from build123d import *

# Parameters (mm, degrees)
SKETCH2_R           = 2
BOSS_EXTRUDE1_DEPTH = 6.7


with BuildPart() as part:
    # Sketch2 → Boss-Extrude1 (new body)
    with BuildSketch(Plane.XY):
        with BuildLine():
            Line((-4.409637173, -1.2), (-3.764514138, -0.899174188))
            ThreePointArc((-3.764514138, -0.899174188), (-3.582420347, -0.728223333), (-3.537232834, -0.482580436))
            ThreePointArc((-3.537232834, -0.482580436), (-3.57, 0), (-3.537232834, 0.482580436))
            ThreePointArc((-3.537232834, 0.482580436), (-3.582420347, 0.728223333), (-3.764514138, 0.899174188))
            Line((-3.764514138, 0.899174188), (-4.409637173, 1.2))
            ThreePointArc((-4.409637173, 1.2), (-4.294395277, 1.563032055), (-4.149323184, 1.915206806))
            Line((-4.149323184, 1.915206806), (-3.461763164, 1.730975654))
            ThreePointArc((-3.461763164, 1.730975654), (-3.212386135, 1.744883974), (-3.019874282, 1.904011377))
            ThreePointArc((-3.019874282, 1.904011377), (-2.734778662, 2.294751767), (-2.399480831, 2.6433675))
            ThreePointArc((-2.399480831, 2.6433675), (-2.276200264, 2.860586849), (-2.305807109, 3.108590435))
            Line((-2.305807109, 3.108590435), (-2.606632921, 3.75371347))
            ThreePointArc((-2.606632921, 3.75371347), (-2.285, 3.957736095), (-1.947494763, 4.134267063))
            Line((-1.947494763, 4.134267063), (-1.539214732, 3.55118275))
            ThreePointArc((-1.539214732, 3.55118275), (-1.339240749, 3.401540677), (-1.089482991, 3.399695106))
            ThreePointArc((-1.089482991, 3.399695106), (-0.619923994, 3.515763678), (-0.13898508, 3.567293533))
            ThreePointArc((-0.13898508, 3.567293533), (0.095079219, 3.654449987), (0.231812692, 3.863462669))
            Line((0.231812692, 3.863462669), (0.416043844, 4.551022689))
            ThreePointArc((0.416043844, 4.551022689), (0.793572172, 4.500571431), (1.165588102, 4.418857814))
            Line((1.165588102, 4.418857814), (1.10354938, 3.709751971))
            ThreePointArc((1.10354938, 3.709751971), (1.160550267, 3.466578694), (1.3506895, 3.304623712))
            ThreePointArc((1.3506895, 3.304623712), (1.785, 3.091710692), (2.186543334, 2.822043275))
            ThreePointArc((2.186543334, 2.822043275), (2.421870079, 2.738355361), (2.660964759, 2.810577782))
            Line((2.660964759, 2.810577782), (3.244049071, 3.218857814))
            ThreePointArc((3.244049071, 3.218857814), (3.500823105, 2.937539376), (3.73327934, 2.635815883))
            Line((3.73327934, 2.635815883), (3.229950472, 2.132487015))
            ThreePointArc((3.229950472, 2.132487015), (3.117306916, 1.909566013), (3.158859362, 1.663282156))
            ThreePointArc((3.158859362, 1.663282156), (3.354702656, 1.221011912), (3.488963822, 0.756327606))
            ThreePointArc((3.488963822, 0.756327606), (3.615441013, 0.540953828), (3.845021841, 0.442592316))
            Line((3.845021841, 0.442592316), (4.554127684, 0.380553593))
            ThreePointArc((4.554127684, 0.380553593), (4.57, 0), (4.554127684, -0.380553593))
            Line((4.554127684, -0.380553593), (3.845021841, -0.442592316))
            ThreePointArc((3.845021841, -0.442592316), (3.615441013, -0.540953828), (3.488963822, -0.756327606))
            ThreePointArc((3.488963822, -0.756327606), (3.354702656, -1.221011912), (3.158859362, -1.663282156))
            ThreePointArc((3.158859362, -1.663282156), (3.117306916, -1.909566013), (3.229950472, -2.132487015))
            Line((3.229950472, -2.132487015), (3.73327934, -2.635815883))
            ThreePointArc((3.73327934, -2.635815883), (3.500823105, -2.937539376), (3.244049071, -3.218857814))
            Line((3.244049071, -3.218857814), (2.660964759, -2.810577782))
            ThreePointArc((2.660964759, -2.810577782), (2.421870079, -2.738355361), (2.186543334, -2.822043275))
            ThreePointArc((2.186543334, -2.822043275), (1.785, -3.091710692), (1.3506895, -3.304623712))
            ThreePointArc((1.3506895, -3.304623712), (1.160550267, -3.466578694), (1.10354938, -3.709751971))
            Line((1.10354938, -3.709751971), (1.165588102, -4.418857814))
            ThreePointArc((1.165588102, -4.418857814), (0.793572172, -4.500571431), (0.416043844, -4.551022689))
            Line((0.416043844, -4.551022689), (0.231812692, -3.863462669))
            ThreePointArc((0.231812692, -3.863462669), (0.095079219, -3.654449987), (-0.13898508, -3.567293533))
            ThreePointArc((-0.13898508, -3.567293533), (-0.619923994, -3.515763678), (-1.089482991, -3.399695106))
            ThreePointArc((-1.089482991, -3.399695106), (-1.339240749, -3.401540677), (-1.539214732, -3.55118275))
            Line((-1.539214732, -3.55118275), (-1.947494763, -4.134267063))
            ThreePointArc((-1.947494763, -4.134267063), (-2.285, -3.957736095), (-2.606632921, -3.75371347))
            Line((-2.606632921, -3.75371347), (-2.305807109, -3.108590435))
            ThreePointArc((-2.305807109, -3.108590435), (-2.276200264, -2.860586849), (-2.399480831, -2.6433675))
            ThreePointArc((-2.399480831, -2.6433675), (-2.734778662, -2.294751767), (-3.019874282, -1.904011377))
            ThreePointArc((-3.019874282, -1.904011377), (-3.212386135, -1.744883974), (-3.461763164, -1.730975654))
            Line((-3.461763164, -1.730975654), (-4.149323184, -1.915206806))
            ThreePointArc((-4.149323184, -1.915206806), (-4.294395277, -1.563032055), (-4.409637173, -1.2))
        make_face()
        Circle(SKETCH2_R, mode=Mode.SUBTRACT)
    extrude(amount=BOSS_EXTRUDE1_DEPTH)


solid = part.part
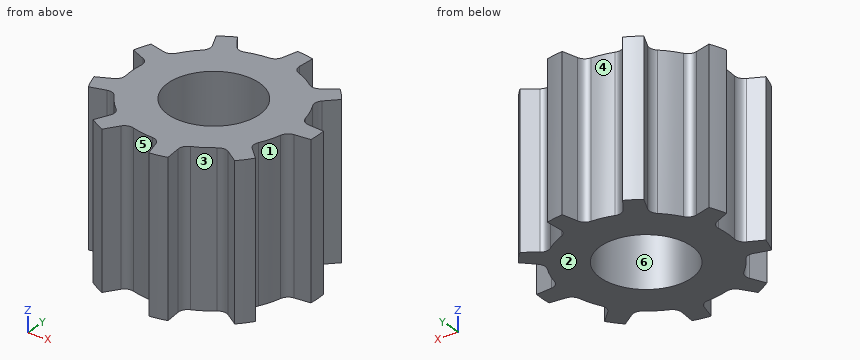
Geometry check sheet. Reference: the model listing, model coordinates, mm. Face numbers are marked on the shaded views. A direction names the side the tool comes from. Round coordinates to 2 decimals unless told otherwise and drop trailing zeros. Order: outer loops, then holes, each group sorted by start corner. A loop starts at its lowest first (then second) coordinate and runs counter-clockwise, first axis right, second up. Notation, with made-up numbers: (38, 13.25) - (65, 13.25) arc R14 ccw to (65, 30.25) - close; hole circle Ø6 at (-39.5, 47.25). An arc over 180 degrees is marked (long way). One line per question, with ' | ' between items. Start each with the question number.
(1) Depth check by flat-ended pin: pin 1 Ø1.5 at (x, z) = (2, 5.5) entering from -Y; pin 2 Ø3 at (x, y) = (0, 0) entering from -Z. Enter the tip coordinate at first touch or a pass-through.
(2) Sectioned sample at B-B on x = 0. Record the cut outline in (y, z), and give its area (3 significant figures).
(3) Release check for a two-part mould opening along Y. For the marked faces 4, 5 and 6 record: released by +Y, released by -Y, zero draft, split by the parting line, or undercut.
(4) Sectioned sample at C-C on x = 4. Record the cut outline in (y, z), and give its area (3 significant figures).
(5) Access from +Z, -Z, +X, -X, +Y, -Y to the whole of each face (thin tool, end or side, straight path). Record for the marked faces 1, 2 and 3.
(6) Sectioned sample at A-A on y = 0. Record the cut outline in (x, z), and give its area (3 significant figures).
(7) Thickness scan on L1, parallel to Y at x = 0, z = 2.25; L2, parallel to X at y = -1.25, z = 3; L3, parallel to X at y = 3, z = 3. Record the ranges inside material, lowest first. Write a range as [from, to].
Conclusion:
1) pin 1: stops at y = -3.36 | pin 2: passes through
2) outline: (-3.6, 0) - (-2, 0) - (-2, 6.7) - (-3.6, 6.7) - close; (2, 0) - (3.6, 0) - (3.6, 6.7) - (2, 6.7) - close | area: 21.4 mm2
3) face 4: released by +Y | face 5: released by -Y | face 6: undercut
4) outline: (-0.43, 0) - (0.43, 0) - (0.43, 6.7) - (-0.43, 6.7) - close | area: 5.75 mm2
5) face 1: +Z, -Z, +X | face 2: -Z, +X, -X, +Y, -Y | face 3: +Z, -Z, -Y
6) outline: (-3.57, 0) - (-2, 0) - (-2, 6.7) - (-3.57, 6.7) - close; (2, 0) - (4.57, 0) - (4.57, 6.7) - (2, 6.7) - close | area: 27.7 mm2
7) L1: y = [-3.6, -2], [2, 3.6] | L2: x = [-4.4, -1.56], [1.56, 3.34] | L3: x = [-2.27, 1.94], [2.93, 3.45]
